Part model, mm, in its own coordinate system. A direction names the side the tool comes from. Give positions to 0.01 mm unless a question says otherwise; leave off trailing zeros. Order: outer loops, then holes, each group sorted by start corner. A loop starts at its lowest first (then second) coordinate and runs counter-clockwise, first axis right, second up. Notation, with made-up numbers: M -25,72.25 L 11,72.25 A21 cw 11,94.25 Z; hole C 43.25,86.5 d3. An arc over 180 degrees is marked long. Answer as a JSON object with one key per item and string values.
from build123d import *

# Parameters (mm, degrees)
SKETCH1_R           = 2
SKETCH1_R_2         = 2.99
SKETCH1_R_3         = 1.7
BOSS_EXTRUDE1_DEPTH = 10
FILLET1_R           = 2
FILLET2_R           = 3
SKETCH1_4_R         = 2.99
CUT_EXTRUDE3_DEPTH  = 5.07
SKETCH1_5_R         = 2
CUT_EXTRUDE4_DEPTH  = 2.48
CUT_EXTRUDE5_DEPTH  = 3
SKETCH1_7_R         = 1.7
CUT_EXTRUDE6_DEPTH  = 10
SKETCH4_R           = 1.25
CUT_EXTRUDE7_DEPTH  = 10
SKETCH5_R           = 2.725
CUT_EXTRUDE8_DEPTH  = 2.8


with BuildPart() as part:
    # Sketch1 → Boss-Extrude1 (new body)
    with BuildSketch(Plane(origin=(0, 0, 0), x_dir=(1, 0, 0), z_dir=(0, 1, 0))):
        with BuildLine():
            ThreePointArc((-9.409245094, 8.977987014), (-7.849239736, 9.28), (-6.289234378, 8.977987014))
            ThreePointArc((-6.289234378, 8.977987014), (-3.835653376, 8.254222737), (-1.289234378, 8.01))
            Line((-1.289234378, 8.01), (38.12, 8.01))
            Line((38.12, 8.01), (38.12, -3.81))
            Line((38.12, -3.81), (28.478275237, -3.81))
            Line((28.478275237, -3.81), (26.178275237, 0))
            Line((26.178275237, 0), (-26.178275237, 0))
            Line((-26.178275237, 0), (-28.478275237, -3.81))
            Line((-28.478275237, -3.81), (-38.12, -3.81))
            Line((-38.12, -3.81), (-38.12, 8.01))
            Line((-38.12, 8.01), (-14.409245094, 8.01))
            ThreePointArc((-14.409245094, 8.01), (-11.862826096, 8.254222737), (-9.409245094, 8.977987014))
        make_face()
        with Locations((20, 4.005)):
            Circle(SKETCH1_R, mode=Mode.SUBTRACT)
        with Locations((-20, 4.005)):
            Circle(SKETCH1_R, mode=Mode.SUBTRACT)
        with Locations((-32.12, 1.98)):
            Circle(SKETCH1_R_2, mode=Mode.SUBTRACT)
        with Locations((32.12, 1.98)):
            Circle(SKETCH1_R_2, mode=Mode.SUBTRACT)
        with Locations((-7.849239736, 5.1)):
            Circle(SKETCH1_R_3, mode=Mode.SUBTRACT)
        with BuildLine():
            ThreePointArc((9.912105026, 2.53), (12.127105026, 4.745), (9.912105026, 6.96))
            Line((9.912105026, 6.96), (3.992105026, 6.96))
            ThreePointArc((3.992105026, 6.96), (1.777105026, 4.745), (3.992105026, 2.53))
            Line((3.992105026, 2.53), (9.912105026, 2.53))
        make_face(mode=Mode.SUBTRACT)
        with Locations((-20, 4.005)):
            Circle(SKETCH1_R)
        with Locations((-7.849239736, 5.1)):
            Circle(SKETCH1_R_3)
        with Locations((-32.12, 1.98)):
            Circle(SKETCH1_R_2)
        with BuildLine():
            Line((3.992105026, 2.53), (9.912105026, 2.53))
            ThreePointArc((9.912105026, 2.53), (12.127105026, 4.745), (9.912105026, 6.96))
            Line((9.912105026, 6.96), (3.992105026, 6.96))
            ThreePointArc((3.992105026, 6.96), (1.777105026, 4.745), (3.992105026, 2.53))
        make_face()
        with Locations((20, 4.005)):
            Circle(SKETCH1_R)
        with Locations((32.12, 1.98)):
            Circle(SKETCH1_R_2)
    extrude(amount=-BOSS_EXTRUDE1_DEPTH)

    # Fillet1
    fillet1_edges = [part.edges().sort_by_distance(p)[0] for p in [
        (26.178275237, -5, 0),
        (-26.178275237, -5, 0),
    ]]
    fillet(fillet1_edges, radius=FILLET1_R)

    # Fillet2
    fillet2_edges = [part.edges().sort_by_distance(p)[0] for p in [
        (28.478275237, -5, 3.81),
        (-28.478275237, -5, 3.81),
    ]]
    fillet(fillet2_edges, radius=FILLET2_R)

    # Sketch1<4> → Cut-Extrude3 (cut)
    with BuildSketch(Plane(origin=(0, 0, 0), x_dir=(1, 0, 0), z_dir=(0, 1, 0))):
        with Locations((32.12, 1.98)):
            Circle(SKETCH1_4_R)
        with Locations((-32.12, 1.98)):
            Circle(SKETCH1_4_R)
    extrude(amount=-CUT_EXTRUDE3_DEPTH, mode=Mode.SUBTRACT)

    # Sketch1<5> → Cut-Extrude4 (cut)
    with BuildSketch(Plane(origin=(0, 0, 0), x_dir=(1, 0, 0), z_dir=(0, 1, 0))):
        with Locations((-20, 4.005)):
            Circle(SKETCH1_5_R)
        with Locations((20, 4.005)):
            Circle(SKETCH1_5_R)
    extrude(amount=-CUT_EXTRUDE4_DEPTH, mode=Mode.SUBTRACT)

    # Sketch1<6> → Cut-Extrude5 (cut)
    with BuildSketch(Plane(origin=(0, 0, 0), x_dir=(1, 0, 0), z_dir=(0, 1, 0))):
        with BuildLine():
            Line((3.992105026, 2.53), (9.912105026, 2.53))
            ThreePointArc((9.912105026, 2.53), (12.127105026, 4.745), (9.912105026, 6.96))
            Line((9.912105026, 6.96), (3.992105026, 6.96))
            ThreePointArc((3.992105026, 6.96), (1.777105026, 4.745), (3.992105026, 2.53))
        make_face()
    extrude(amount=-CUT_EXTRUDE5_DEPTH, mode=Mode.SUBTRACT)

    # Sketch1<7> → Cut-Extrude6 (cut)
    with BuildSketch(Plane(origin=(0, 0, 0), x_dir=(1, 0, 0), z_dir=(0, 1, 0))):
        with Locations((-7.849239736, 5.1)):
            Circle(SKETCH1_7_R)
    extrude(amount=-CUT_EXTRUDE6_DEPTH, mode=Mode.SUBTRACT)

    # Sketch4 → Cut-Extrude7 (cut)
    with BuildSketch(Plane(origin=(0, 0, 0), x_dir=(1, 0, 0), z_dir=(0, 1, 0))):
        with Locations((-20, 4.005)):
            Circle(SKETCH4_R)
        with Locations((20, 4.005)):
            Circle(SKETCH4_R)
    extrude(amount=-CUT_EXTRUDE7_DEPTH, mode=Mode.SUBTRACT)

    # Sketch5 → Cut-Extrude8 (cut)
    with BuildSketch(Plane.XZ.offset(10)):
        with Locations((20, -4.005)):
            Circle(SKETCH5_R)
        with Locations((-20, -4.005)):
            Circle(SKETCH5_R)
    extrude(amount=-CUT_EXTRUDE8_DEPTH, mode=Mode.SUBTRACT)


solid = part.part
1. Probe line 1 along X through (y, z) = (-2.25, -1.75); line 2 along Z through (x, y) = (32.12, -2.9); line 3 along Z through (x, y) = (20, -9.05). List the from-to ranges inside material, lowest first.
Worked answers:
{"line 1": "x = -38.12 to -35.1, -29.14 to 29.14, 35.1 to 38.12", "line 2": "z = -8.01 to -4.97, 1.01 to 3.81", "line 3": "z = -8.01 to -6.73, -1.28 to 0"}
2. Which spindle directions (+Z, -Z, +X, -X, +Y, -Y) get a long thin tool onto all of the face, cutting with end or side? Do faces 5 (the flat face through (21, -7.2, -5)), 6 (the flat face through (1, 0, -4)), 7 (the flat face through (27.188, -4.93, 1.673)), 8 (the flat face through (7, -1, -6.96)). Say none if no direction does.
Worked answers:
{"face 5": "-Y", "face 6": "+Z, -Z, +X, -X, +Y", "face 7": "+Z, +Y, -Y", "face 8": "+Y"}
3. Cut at D-D on y = -6. State how many separate pieces and enclosed holes the cut face has, plus the area to 3 significant figures.
Worked answers:
{"separate pieces": "1", "enclosed holes": "3", "area": "680 mm^2"}
4. Cut at B-B on y = -1.75. Give the cut face in (x, z) (1 decimal).
Worked answers:
{"outline": "M -38.1,-8 L -14.4,-8 A13.4 cw -9.4,-9 A4.2 ccw -6.3,-9 A13.4 cw -1.3,-8 L 38.1,-8 L 38.1,3.8 L 30.2,3.8 A3 ccw 27.6,2.4 L 26.8,1 A2 cw 25,0 L -25,0 A2 cw -26.8,1 L -27.6,2.4 A3 ccw -30.2,3.8 L -38.1,3.8 Z; hole C -32.1,-2 d6; hole C -20,-4 d4; hole C -7.8,-5.1 d3.4; hole M 4,-7 L 9.9,-7 A2.2 ccw 9.9,-2.5 L 4,-2.5 A2.2 ccw Z; hole C 20,-4 d4; hole C 32.1,-2 d6"}
5. Cut at C-C on x = 32.12. Give the cut face in (y, z).
Worked answers:
{"outline": "M -10,-8.01 L 0,-8.01 L 0,-4.97 L -5.07,-4.97 L -5.07,1.01 L 0,1.01 L 0,3.81 L -10,3.81 Z"}
6. Pin check, flat tips, straight feed: P1, Ø2, axis at x = 28.5, y = -7.5, coming from the +Z side; P2, Ø5.5, axis at x = -32.12, z = -1.98, coming from the +Y side; P3, Ø1.6, axis at x = -19.5, z = -5, coming from the -Y side. Stop position of each tip, or through.
Worked answers:
{"P1": "stops at z = 3.73", "P2": "stops at y = -5.07", "P3": "stops at y = -7.2"}
7. Two-plate mould, pull along Z, no slides. Class faces 1 (the cylindrical face through (17.838, -8.62, -5.663)), 2 (the flat face through (1, -10, -4)), 3 (the cylindrical face through (-28.678, -5.07, 3.412)), 4 (the flat face through (7, -1, -2.53)): +Z half, -Z half, draft (parallel to the pull), parting line (faces both ways), or undercut.
Worked answers:
{"face 1": "undercut", "face 2": "draft", "face 3": "+Z half", "face 4": "undercut"}
8. Cut at A-A on x = -20. Give the cut face in (y, z) (3 decimals).
Worked answers:
{"outline": "M -10,-8.01 L 0,-8.01 L 0,-6.005 L -2.48,-6.005 L -2.48,-5.255 L -7.2,-5.255 L -7.2,-6.73 L -10,-6.73 Z; M -10,-1.28 L -7.2,-1.28 L -7.2,-2.755 L -2.48,-2.755 L -2.48,-2.005 L 0,-2.005 L 0,0 L -10,0 Z"}
